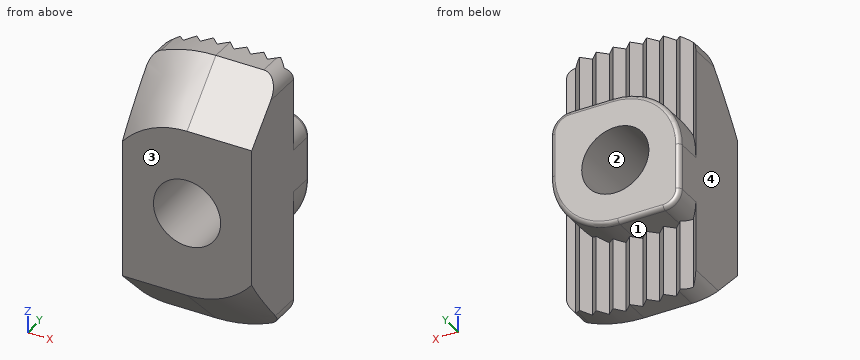
```python
from build123d import *

# Parameters (mm, degrees)
EXTRUDE1_DEPTH          = 4.5
CUT_EXTRUDE1_DEPTH      = 8
CUT_EXTRUDE1_DEPTH_BACK = 8
EXTRUDE2_DEPTH          = 6.00039994
CUT_EXTRUDE2_DEPTH      = 4
CUT_EXTRUDE2_DEPTH_BACK = 4
CUT_REVOLVE1_ANGLE      = 60
CUT_REVOLVE2_ANGLE      = 60
SKETCH9_R               = 2.48793
CUT_EXTRUDE3_DEPTH      = 7.00040004
FILLET4_R               = 0.25
SKETCH10_R              = 2.48793
EXTRUDE3_DEPTH          = 6.0004
SKETCH12_R              = 2
CUT_EXTRUDE4_DEPTH      = 7.00040004


with BuildPart() as part:
    # Sketch1 → Extrude1 (new body)
    with BuildSketch(Plane(origin=(0, 0, 0), x_dir=(1, 0, 0), z_dir=(0, 1, 0))):
        with BuildLine():
            Line((0, -8), (2.85, -8))
            ThreePointArc((2.85, -8), (3.557106781, -7.707106781), (3.85, -7))
            Line((3.85, -7), (3.85, 6.393551439))
            ThreePointArc((3.85, 6.393551439), (3.688791661, 6.938003962), (3.2571429, 7.306915911))
            ThreePointArc((3.2571429, 7.306915911), (1.66503344, 7.824810774), (0, 8))
            Line((0, 8), (-2.85, 8))
            ThreePointArc((-2.85, 8), (-3.557106781, 7.707106781), (-3.85, 7))
            Line((-3.85, 7), (-3.85, -6.393551439))
            ThreePointArc((-3.85, -6.393551439), (-3.688791661, -6.938003962), (-3.2571429, -7.306915911))
            ThreePointArc((-3.2571429, -7.306915911), (-1.66503344, -7.824810774), (0, -8))
        make_face()
    extrude(amount=EXTRUDE1_DEPTH)

    # Sketch2 → Cut-Extrude1 (cut, two sides)
    with BuildSketch(Plane.XY) as cut_extrude1_sk:
        Polygon((-4, 4.5), (-3.5, 4), (-3, 4.5), (-2.5, 4), (-2, 4.5), (-1.5, 4), (-1, 4.5), (-0.5, 4), (0, 4.5), (0.5, 4), (1, 4.5), (1.5, 4), (2, 4.5), (2.5, 4), (3, 4.5), (3.5, 4), (4, 4.5), (4, 5.5), (-4, 5.5), align=None)
    extrude(amount=CUT_EXTRUDE1_DEPTH, mode=Mode.SUBTRACT)
    extrude(cut_extrude1_sk.sketch, amount=-CUT_EXTRUDE1_DEPTH_BACK, mode=Mode.SUBTRACT)

    # Sketch3 → Extrude2 (add)
    with BuildSketch(Plane(origin=(0, 0, 0), x_dir=(1, 0, 0), z_dir=(0, 1, 0))):
        with BuildLine():
            Line((0.15, -3.85), (2.693303618, -3.85))
            ThreePointArc((2.693303618, -3.85), (3.511211473, -3.511211473), (3.85, -2.693303618))
            Line((3.85, -2.693303618), (3.85, -0.15))
            ThreePointArc((3.85, -0.15), (2.678427125, 2.678427125), (-0.15, 3.85))
            Line((-0.15, 3.85), (-2.85, 3.85))
            ThreePointArc((-2.85, 3.85), (-3.557106781, 3.557106781), (-3.85, 2.85))
            Line((-3.85, 2.85), (-3.85, 0.15))
            ThreePointArc((-3.85, 0.15), (-2.678427125, -2.678427125), (0.15, -3.85))
        make_face()
    extrude(amount=EXTRUDE2_DEPTH)

    # Sketch4 → Cut-Extrude2 (cut, two sides)
    with BuildSketch(Plane(origin=(0, 0, 0), x_dir=(0, 0, -1), z_dir=(1, 0, 0))) as cut_extrude2_sk:
        Polygon((-9, -1), (9, -1), (9, 4), (5, 0), (-5, 0), (-9, 4), align=None)
    extrude(amount=CUT_EXTRUDE2_DEPTH, mode=Mode.SUBTRACT)
    extrude(cut_extrude2_sk.sketch, amount=-CUT_EXTRUDE2_DEPTH_BACK, mode=Mode.SUBTRACT)

    # Sketch5 → Cut-Revolve1 (revolve, cut)
    with BuildSketch(Plane(origin=(0, 0, 0), x_dir=(0, 0, -1), z_dir=(1, 0, 0))):
        Polygon((0, -1), (-9, -1), (-9, 3), (-8, 3), (-5, 0), (0, 0), align=None)
    revolve(axis=Axis((0, 3, 0), (0, -1, 0)), revolution_arc=CUT_REVOLVE1_ANGLE, mode=Mode.SUBTRACT)

    # Sketch6 → Cut-Revolve2 (revolve, cut)
    with BuildSketch(Plane(origin=(0, 0, 0), x_dir=(0, 0, -1), z_dir=(1, 0, 0))):
        Polygon((0, 0), (5, 0), (8, 3), (9, 3), (9, -1), (0, -1), align=None)
    revolve(axis=Axis((0, -1, 0), (0, -1, 0)), revolution_arc=CUT_REVOLVE2_ANGLE, mode=Mode.SUBTRACT)

    # Sketch9 → Cut-Extrude3 (cut, through all)
    with BuildSketch(Plane(origin=(0, 6.00039994, 0), x_dir=(1, 0, 0), z_dir=(0, 1, 0))):
        Circle(SKETCH9_R)
    extrude(amount=-CUT_EXTRUDE3_DEPTH, mode=Mode.SUBTRACT)

    # Fillet4
    fillet4_edges = [part.edges().sort_by_distance(p)[0] for p in [
        (-2.678427125, 6.00039994, 2.678427125),
        (1.421651809, 6.00039994, 3.85),
        (3.511211473, 6.00039994, 3.511211473),
        (3.85, 6.00039994, 1.421651809),
        (2.678427125, 6.00039994, -2.678427125),
        (-1.5, 6.00039994, -3.85),
        (-3.557106781, 6.00039994, -3.557106781),
        (-3.85, 6.00039994, -1.5),
    ]]
    fillet(fillet4_edges, radius=FILLET4_R)

    # Sketch10 → Extrude3 (add)
    with BuildSketch(Plane(origin=(0, 6.00039994, 0), x_dir=(1, 0, 0), z_dir=(0, 1, 0))):
        Circle(SKETCH10_R)
    extrude(amount=-EXTRUDE3_DEPTH)

    # Sketch12 → Cut-Extrude4 (cut, through all)
    with BuildSketch(Plane(origin=(0, 6.00039994, 0), x_dir=(1, 0, 0), z_dir=(0, 1, 0))):
        Circle(SKETCH12_R)
    extrude(amount=-CUT_EXTRUDE4_DEPTH, mode=Mode.SUBTRACT)


solid = part.part
```
The listing builds one solid part. Answer for the finished solid, in the listing's coordinates (mm). Face numbers are marked on the shaded views. Coordinates: 2 decimals unless noted, no trailing zeros. Write each loop counter-clockwise with the first axis right and the second up, starting at its lowest first coordinate (ties: lowest second). Pieces come first, ordered by that corner, then holes. Notation, with made-up numbers: (25.25, 46.5) - (69.25, 46.5) arc R18 cw to (69.25, 74.5) - close; hole circle Ø1 at (75.25, 53). An arc over 180 degrees is marked (long way). Return JSON: item names as keys, results as strings. Group by question number.
Q1. For a pull along X with two mould halves and no side action, classify the marked faces 1, 2, 3 and 4 as +X half, -X half, draft (parallel to the pull), parting line (faces both ways), or undercut.
Q2. The part is cut by section B-B on y = 2.25. Write down the section's boundary in (x, z), and give its area (3 significant figures).
Q3. The part is cut by section A-A on y = 3.25. Write down the section's boundary in (x, z).
Q4. Flat-ended cylindrical pins translate along their axes: pin 1 Ø1 at (x, z) = (1, 0) entering from -Y; pin 2 Ø2 at (x, y) = (-2, 1.5) entering from +Z. Find the tip coordinate at first contact, or state that the pin passes through.
Q5. Find the intervals of material crossed by line 1 along X through (y, z) = (3, 0); line 2 along X through (y, z) = (5.5, 3), in increasing order. Write a range as [from, to].
Evaluation:
{
 "1": {"face 1": "undercut", "face 2": "undercut", "face 3": "draft", "face 4": "-X half"},
 "2": {"outline": "(-3.85, -7) arc R1 ccw to (-3.82, -7.25) - (0, -7.25) arc R7.25 ccw to (3.85, -6.14) - (3.85, 7) arc R1 ccw to (3.82, 7.25) - (0, 7.25) arc R7.25 ccw to (-3.85, 6.14) - close; hole circle Ø4 at (0, 0)", "area": "96.3 mm2"},
 "3": {"outline": "(-3.85, -7) arc R1 ccw to (-2.85, -8) - (0, -8) arc R8 ccw to (3.26, -7.31) arc R1 ccw to (3.85, -6.39) - (3.85, 7) arc R1 ccw to (2.85, 8) - (0, 8) arc R8 ccw to (-3.26, 7.31) arc R1 ccw to (-3.85, 6.39) - close; hole circle Ø4 at (0, 0)"},
 "4": {"pin 1": "passes through", "pin 2": "stops at z = 7.26"},
 "5": {"line 1": "x = [-3.85, -2], [2, 3.85]", "line 2": "x = [-2.32, 3.81]"}
}
